```python
from build123d import *

# Parameters (mm, degrees)
F1_DEPTH      = 50
F2_R          = 1.25
F3_DEPTH      = 32.901
F2_R_2        = 3.5
F4_DEPTH      = 2.1
F4_DEPTH_BACK = 10
F5_T1_DEPTH   = 75


# Not quite as in the source:
# - a fillet or chamfer that OpenCascade refuses, or shapes differently, is made with other operations: its cross-section is extruded or revolved along the edge and cut away or added


with BuildPart() as f1:
    # F0 (on Top) → F1 (new body)
    with BuildSketch(Plane.XY):
        with BuildLine():
            ThreePointArc((0, 4), (-1.1715728753, 1.1715728753), (-4, 0))
            Line((-4, 0), (-26.8, 0))
            ThreePointArc((-26.8, 0), (-29.6284271247, 1.1715728753), (-30.8, 4))
            Line((-30.8, 4), (-30.8, 15))
            Line((-30.8, 15), (-32.9, 15))
            Line((-32.9, 15), (-32.9, -2.1))
            Line((-32.9, -2.1), (2.1, -2.1))
            Line((2.1, -2.1), (2.1, 45))
            Line((2.1, 45), (-12.9, 45))
            Line((-12.9, 45), (-12.9, 42.9))
            Line((-12.9, 42.9), (-4, 42.9))
            ThreePointArc((-4, 42.9), (-1.1715728753, 41.7284271247), (0, 38.9))
            Line((0, 38.9), (0, 4))
        make_face()
    extrude(amount=F1_DEPTH)

    # F2 (on Right) → F3 (cut, through all)
    with BuildSketch(Plane.YZ):
        with Locations((5.4, 35)):
            Circle(F2_R)
        with Locations((5.4, 15)):
            Circle(F2_R)
    extrude(amount=-F3_DEPTH, mode=Mode.SUBTRACT)

    # F2 (on Right) → F4 (cut, two sides)
    with BuildSketch(Plane.YZ) as f4_sk:
        with Locations((5.4, 35)):
            Circle(F2_R_2)
        with Locations((5.4, 35)):
            Circle(F2_R, mode=Mode.SUBTRACT)
        with Locations((5.4, 15)):
            Circle(F2_R_2)
        with Locations((5.4, 15)):
            Circle(F2_R, mode=Mode.SUBTRACT)
        with Locations((5.4, 15)):
            Circle(F2_R)
        with Locations((5.4, 35)):
            Circle(F2_R)
    extrude(amount=F4_DEPTH, mode=Mode.SUBTRACT)
    extrude(f4_sk.sketch, amount=-F4_DEPTH_BACK, mode=Mode.SUBTRACT)

    # F5: fillet of radius 5 on 2 edges, made by hand

    # F5_s2 → F5_t1 (cut)
    with BuildSketch(Plane.XY.offset(-12.5)):
        with BuildLine():
            ThreePointArc((2.1, 40), (0.6355339059, 43.5355339059), (-2.9, 45))
            Line((-2.9, 45), (2.1, 45))
            Line((2.1, 45), (2.1, 40))
        make_face()
        with BuildLine():
            ThreePointArc((-2.9, -2.1), (0.6355339059, -0.6355339059), (2.1, 2.9))
            Line((2.1, 2.9), (2.1, -2.1))
            Line((2.1, -2.1), (-2.9, -2.1))
        make_face()
    extrude(amount=F5_T1_DEPTH, mode=Mode.SUBTRACT)


solid = f1.part
```
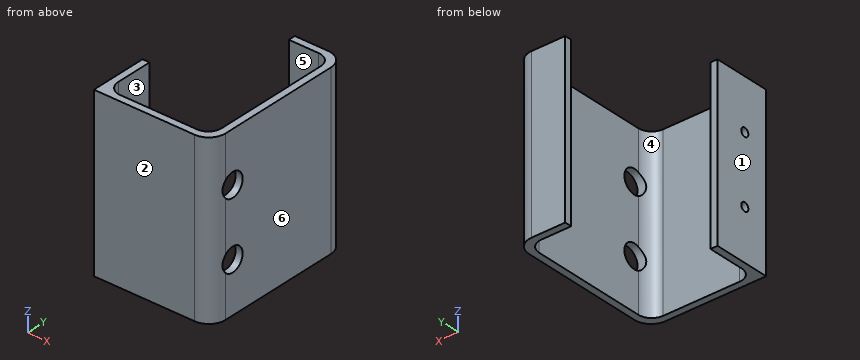
Design review of the part built by this model. Coordinates are the model's own, in mm. Face numbers are marked on the shaded views. A direction names the side the tool comes from. Round coordinates to 2 decimals unless told otherwise and drop trailing zeros. Order: outer loops, then holes, each group sorted by start corner. A loop starts at its lowest first (then second) coordinate and runs counter-clockwise, first axis right, second up. Notation, with made-up numbers: (-34, 75) - (-29, 75) arc R25 cw to (-29, 98) - close; hole circle Ø2 at (-12, 87.5). An arc over 180 degrees is marked (long way). One line per question, with ' | ' between items.
Item 1: Machinability: for the marked faces 4, 5 and 6, which of the approach directions +Z, -Z, +X, -X, +Y, -Y give a long, thin tool a straight path to every point of the face, cutting with its end or side? Answer none if there is none.
Checks:
face 4: +Z, -Z | face 5: +Z, -Z, -X | face 6: +Z, -Z, +X, +Y, -Y
Item 2: Take a section at C-C, the plane z = 15. Write out the cut boundary in (x, y).
Checks:
outline: (-32.9, -2.1) - (-2.9, -2.1) arc R5 ccw to (2, 1.9) - (-0.6, 1.9) arc R4 cw to (-4, 0) - (-26.8, 0) arc R4 cw to (-30.8, 4) - (-30.8, 4.15) - (-32.9, 4.15) - close; (-32.9, 6.65) - (-30.8, 6.65) - (-30.8, 15) - (-32.9, 15) - close; (-12.9, 42.9) - (-4, 42.9) arc R4 cw to (0, 38.9) - (0, 8.9) - (2.1, 8.9) - (2.1, 40) arc R5 ccw to (-2.9, 45) - (-12.9, 45) - close
Item 3: Take a section at B-B, the plane y = 5.4. Write out the cut boundary in (x, z), then the cut area to 3 significant figures.
Checks:
outline: (-32.9, 0) - (-30.8, 0) - (-30.8, 13.75) - (-32.9, 13.75) - close; (-32.9, 16.25) - (-30.8, 16.25) - (-30.8, 33.75) - (-32.9, 33.75) - close; (-32.9, 36.25) - (-30.8, 36.25) - (-30.8, 50) - (-32.9, 50) - close; (0, 0) - (2.1, 0) - (2.1, 11.5) - (0, 11.5) - close; (0, 18.5) - (2.1, 18.5) - (2.1, 31.5) - (0, 31.5) - close; (0, 38.5) - (2.1, 38.5) - (2.1, 50) - (0, 50) - close | area: 170 mm²
Item 4: Draft analysis for pull direction X (two halves, no side actions). For the marked faces 1, 2 and 3, state which applies: +X half, -X half, draft (parallel to the pull), parting line (faces both ways), or undercut.
Checks:
face 1: -X half | face 2: draft | face 3: undercut
Item 5: Wall thickness on line 1 (X direction, y = 9, z = 23.5); line 2 (Z direction, x = 0.9, y = 5.4); line 3 (Y direction, x = -23, z = 31): over which ranges is each line inside the solid? List them lowest first. Write a range as [from, to].
Checks:
line 1: [-32.9, -30.8], [0, 2.1] | line 2: [0, 11.5], [18.5, 31.5], [38.5, 50] | line 3: [-2.1, 0]
Item 6: Take a section at A-A, the plane x = -10. Write out the cut boundary in (y, z).
Checks:
outline: (-2.1, 0) - (0, 0) - (0, 50) - (-2.1, 50) - close; (42.9, 0) - (45, 0) - (45, 50) - (42.9, 50) - close
Item 7: Take a section at D-D, the plane z = 27. Write out the cut boundary in (x, y).
Checks:
outline: (-32.9, -2.1) - (-2.9, -2.1) arc R5 ccw to (2.1, 2.9) - (2.1, 40) arc R5 ccw to (-2.9, 45) - (-12.9, 45) - (-12.9, 42.9) - (-4, 42.9) arc R4 cw to (0, 38.9) - (0, 4) arc R4 cw to (-4, 0) - (-26.8, 0) arc R4 cw to (-30.8, 4) - (-30.8, 15) - (-32.9, 15) - close
Item 8: For P1, Ø6, axis at x = -12, y = 37, coming from the -Z side; P2, Ø2, axis at y = 20, z = 25.5, coming from the -X side; P3, Ø2.5, axis at x = -32, z = 36.5, coming from the +Y side; P4, Ø0.6, axis at y = 44, z = 33.5, coming from the -X side, all flat-tipped, find the tip position at first contact; note any pin that passes through.
Checks:
P1: through | P2: x = 0 | P3: y = 15 | P4: x = -12.9
